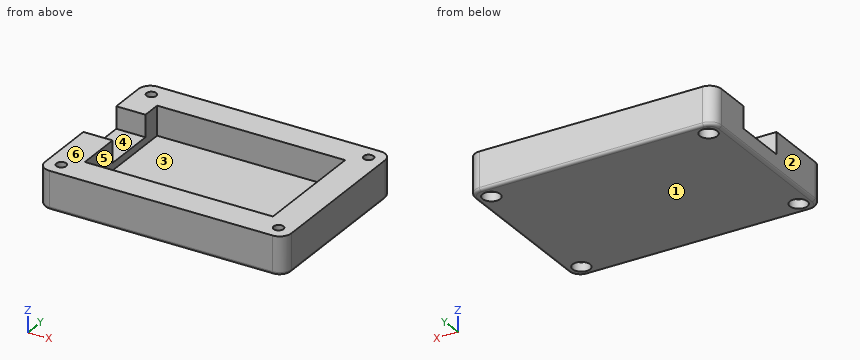
Autodesk Fusion 360 part; units mm, degrees
sketch "Sketch1" plane through (0, 0, 0) normal (0, 0, 1) x (1, 0, 0) in component "Hackpad"
  line L0 (0, 0) -> (64.4, 0)
  line L1 (64.4, 0) -> (64.4, -40.6)
  line L2 (64.4, -40.6) -> (0, -40.6)
  line L3 (0, -40.6) -> (0, 0)
  line L4 (74.4, -50.6) -> (-10, -50.6)
  line L5 (-10, -50.6) -> (-10, 10)
  line L6 (-10, 10) -> (74.4, 10)
  line L7 (74.4, 10) -> (74.4, -50.6)
  circle A0 centre (-5, 5) radius 1.7
  circle A1 centre (69.4, 5) radius 1.7
  circle A2 centre (69.4, -45.6) radius 1.7
  circle A3 centre (-5, -45.6) radius 1.7
  circle A4 centre (-5, 5) radius 3
  circle A5 centre (69.4, 5) radius 3
  circle A6 centre (69.4, -45.6) radius 3
  circle A7 centre (-5, -45.6) radius 3
  dimension "d1" = 40.6
  dimension "d2" = 64.4
  dimension "d3" = -10
  dimension "d4" = 3.4
  dimension "d5" = 3.4
  dimension "d6" = 3.4
  dimension "d7" = 3.4
  dimension "d8" = 5
  dimension "d9" = 5
  dimension "d10" = 5
  dimension "d11" = 5
  dimension "d12" = 5
  dimension "d13" = 5
  dimension "d14" = 5
  dimension "d15" = 5
  dimension "d16" = 6
  dimension "d17" = 6
  dimension "d18" = 6
  dimension "d19" = 6
extrude "Extrude1" add sketch "Sketch1" along normal blind 9.9 from surface at 3.1 contours A4 | A5 | A6 | A7 makes body 1 at (70.2125, 7.8879, 9.7) makes body 2 at (70.2125, -42.7121, 9.7) makes body 3 at (-2.0037, 4.8505, 9.7) makes body 4 at (-2.0037, -45.7495, 9.7) in component "Hackpad"
extrude "Extrude2" add sketch "Sketch1" along normal blind 13 contours L4 L5 L6 L7 bodies 1 2 3 4 in component "Hackpad"
extrude "Extrude3" add sketch "Sketch1" along normal blind 3 contours L0 L1 L2 L3 bodies 1 in component "Hackpad"
sketch "Sketch2" plane through (0, 0, 13) normal (0, 0, 1) x (-1, 0, 0) in component "Hackpad"
  circle A0 centre (-69.4, -5) radius 1.7
  circle A1 centre (5, 45.6) radius 1.7
  line L0 (-64.4, 40.6) -> (0, 40.6)
  line L1 (0, 40.6) -> (0, 0)
  line L2 (0, 0) -> (-64.4, 0)
  line L3 (-64.4, 0) -> (-64.4, 40.6)
  line L4 (-74.4, -10) -> (10, -10)
  line L5 (10, -10) -> (10, 50.6)
  line L6 (10, 50.6) -> (-74.4, 50.6)
  line L7 (-74.4, 50.6) -> (-74.4, -10)
  circle A2 centre (-69.4, 45.6) radius 1.7
  circle A3 centre (5, -5) radius 1.7
  line L8 (10, 6.55) -> (0, 6.55)
  line L9 (0, 6.55) -> (0, 25.05)
  line L10 (0, 25.05) -> (10, 25.05)
  line L11 (10, 25.05) -> (10, 6.55)
  line L12 (-74.4, 50.6) -> (10, 50.6)
  dimension "d27" = 18.5
  dimension "d28" = 25.55
extrude "Extrude4" cut sketch "Sketch2" against normal blind 7.5 contours L1 L5 L8 L9 L10 L11 bodies 1 in component "Hackpad"
fillet "Fillet1" radius 4 4 edges at (-10, -50.6, 6.5) (74.4, -50.6, 6.5) (74.4, 10, 6.5) (-10, 10, 6.5) on bodies 1 in component "Hackpad"
fillet "Fillet2" radius 1 8 edges at (-8.8284, 8.8284, 0) (32.2, 10, 0) (73.2284, 8.8284, 0) (74.4, -20.3, 0) (73.2284, -49.4284, 0) (32.2, -50.6, 0) (-8.8284, -49.4284, 0) (-10, -20.3, 0) on bodies 1 in component "Hackpad"
component "Hackpad" placed x (1, 0, 0) y (0, 1, 0) z (0, 0, 1) at (0, 0, 0)
equation "d1 = 39.6 mm + 1 mm"
equation "d2 = 63.4 mm + 1 mm"
equation "d28 = 19.8 mm + 5.75 mm"
The model under review builds one solid part; all positions refer to its coordinate system, in mm. Face numbers are marked on the shaded views. A direction names the side the tool comes from. Give positions to 0.01 mm unless a question says otherwise; leave off trailing zeros. Write each loop counter-clockwise with the first axis right and the second up, starting at its lowest first coordinate (ties: lowest second). Pieces come first, ordered by that corner, then holes. Notation, with made-up numbers: M 87,-10 L 120,-10 A27 cw 120,13 Z; hole C -15.75,-13.75 d8. An arc over 180 degrees is marked long. One line per question, with ' | ' between items. Start each with the question number.
Item 1: We need section B-B on z = 9.75. Write out the cut boundary in (x, y).
Item 2: Wall thickness on line 1 (Y direction, x = 69.4, z = 1); line 2 (Y direction, x = 18, z = 9.5); line 3 (Y direction, x = -5, z = 10): over which ranges is each line inside the solid? List them lowest first. Write a range as from..to.
Item 3: We need section C-C on x = 69.4. Write out the cut boundary in (y, z).
Item 4: For pin 1 (2.5 mm diameter, centred on x = 69.4, y = 5, fed in from +Z); pin 2 (1.5 mm diameter, centred on x = 53.5, y = -5, fed in from -Z); pin 3 (11 mm diameter, centred on x = -7, y = -17, fed in from +Z); pin 4 (3 mm diameter, centred on y = -21, z = 8, fed in from -X), all flat-tipped, find the tip position at first contact; note any pin that passes through.
Item 5: For the marked faces 4, 5 and 6, list the 3-axis set-ups (+Z, -Z, +X, -X, +Y, -Y) from which the entire face can be reached by the end or side of a thin tool; tool diameter is ignored.
Item 6: Draft analysis for pull direction X (two halves, no side actions). For the marked faces 1, 2 and 3, state which applies: released by +X, released by -X, zero draft, split by the parting line, or undercut.
Item 7: We need section A-A on y = 5. Write out the cut boundary in (x, z).
Item 8: We need section D-D on y = -10.5. Write out the cut boundary in (x, z), plus the area to 3 significant figures.
Results found:
1) outline: M -10,-46.6 A4 ccw -6,-50.6 L 70.4,-50.6 A4 ccw 74.4,-46.6 L 74.4,6 A4 ccw 70.4,10 L -6,10 A4 ccw -10,6 L -10,-6.55 L 0,-6.55 L 0,0 L 64.4,0 L 64.4,-40.6 L 0,-40.6 L 0,-25.05 L -10,-25.05 Z; hole C -5,-45.6 d3.4; hole C -5,5 d3.4; hole C 69.4,-45.6 d3.4; hole C 69.4,5 d3.4
2) line 1: y = -50.6..-48.6, -42.6..2, 8..10 | line 2: y = -50.6..-40.6, 0..10 | line 3: y = -50.6..-47.3, -43.9..-25.05, -6.55..3.3, 6.7..10
3) outline: M -50.6,1 A1 ccw -49.6,0 L -48.6,0 L -48.6,3.1 L -47.3,3.1 L -47.3,13 L -50.6,13 Z; M -43.9,3.1 L -42.6,3.1 L -42.6,0 L 2,0 L 2,3.1 L 3.3,3.1 L 3.3,13 L -43.9,13 Z; M 6.7,3.1 L 8,3.1 L 8,0 L 9,0 A1 ccw 10,1 L 10,13 L 6.7,13 Z
4) pin 1: passes through | pin 2: stops at z = 0 | pin 3: stops at z = 5.5 | pin 4: stops at x = 64.4
5) face 4: +Z, -X | face 5: +Z | face 6: +Z, +X, -X, +Y, -Y
6) face 1: zero draft | face 2: released by -X | face 3: undercut
7) outline: M -10,1 A1 ccw -9,0 L -8,0 L -8,3.1 L -6.7,3.1 L -6.7,13 L -10,13 Z; M -3.3,3.1 L -2,3.1 L -2,0 L 66.4,0 L 66.4,3.1 L 67.7,3.1 L 67.7,13 L -3.3,13 Z; M 71.1,3.1 L 72.4,3.1 L 72.4,0 L 73.4,0 A1 ccw 74.4,1 L 74.4,13 L 71.1,13 Z
8) outline: M -10,1 A1 ccw -9,0 L 73.4,0 A1 ccw 74.4,1 L 74.4,13 L 64.4,13 L 64.4,3 L 0,3 L 0,5.5 L -10,5.5 Z | area: 378 mm2
